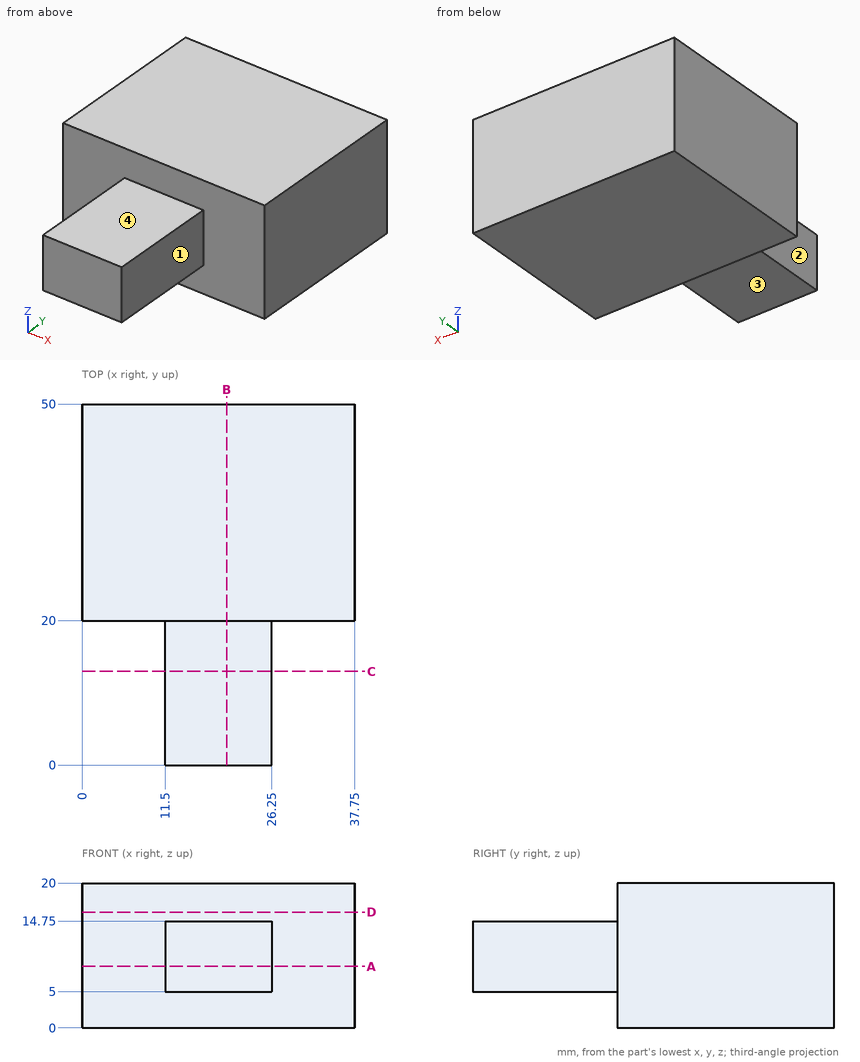
The figure shows three views and two pictorial views of one solid part (mm, origin at its lowest corner). Answer the questions. A direction names the side the tool comes from. Round coordinates to 2 decimals unless told otherwise and drop trailing zeros. Order: outer loops, then holes, each group sorted by start corner. A loop starts at its lowest first (then second) coordinate and runs counter-clockwise, first axis right, second up. Notation, with made-up numbers: M 2,-35.75 L 31,-35.75 A22 cw 31,-18.75 Z; hole C 51,24.25 d10. An arc over 180 degrees is marked long. Answer in a Markdown table with one row per item. Add a question column.
1) Consider line 1 along Z through (x, y) = (25, 13.5); line 2 along Y through (x, z) = (6, 19.25); line 3 along X through (y, z) = (5, 6.25). Determine where each line is inside the solid, lowest interval first. Write a range as from..to.
2) Which of the six approach directions +Z, -Z, +X, -X, +Y, -Y give full straight-line access (tool end or side, diameter ignored) to the marked faces 1, 2, 3 and 4?
3) Flat-ended cylindrical pins translate along their axes: pin 1 Ø2 at (x, y) = (22.5, 6.5) entering from -Z; pin 2 Ø3 at (y, z) = (15, 12) entering from +X; pin 3 Ø10.5 at (y, z) = (6, 8) entering from -X. Find the tip coordinate at first contact, or state that the pin passes through.
4) The part is cut by section B-B on x = 20. Determine the outline of the cut face in (y, z).
5) The part is cut by section D-D on z = 16. Determine the outline of the cut face in (x, y), plus the area to 3 significant figures.
6) The part is cut by section C-C on y = 13. Determine the outline of the cut face in (x, z).
7) The part is cut by section A-A on z = 8.5. Determine the outline of the cut face in (x, y), plus the area to 3 significant figures.
Findings below:
| question | item | result |
|---|---|---|
| 1 | line 1 | z = 5..14.75 |
| 1 | line 2 | y = 20..50 |
| 1 | line 3 | x = 11.5..26.25 |
| 2 | face 1 | +Z, -Z, +X, -Y |
| 2 | face 2 | +Z, -Z, -X, -Y |
| 2 | face 3 | -Z, +X, -X, -Y |
| 2 | face 4 | +Z, +X, -X, -Y |
| 3 | pin 1 | stops at z = 5 |
| 3 | pin 2 | stops at x = 26.25 |
| 3 | pin 3 | stops at x = 11.5 |
| 4 | outline | M 0,5 L 20,5 L 20,0 L 50,0 L 50,20 L 20,20 L 20,14.75 L 0,14.75 Z |
| 5 | outline | M 0,20 L 37.75,20 L 37.75,50 L 0,50 Z |
| 5 | area | 1,130 mm² |
| 6 | outline | M 11.5,5 L 26.25,5 L 26.25,14.75 L 11.5,14.75 Z |
| 7 | outline | M 0,20 L 11.5,20 L 11.5,0 L 26.25,0 L 26.25,20 L 37.75,20 L 37.75,50 L 0,50 Z |
| 7 | area | 1,430 mm² |
